```python
from build123d import *

# Parameters (mm, degrees)
SKETCH1_W           = 40
SKETCH1_H           = 25
BOSS_EXTRUDE1_DEPTH = 14
SKETCH2_R           = 8.15
CUT_EXTRUDE1_DEPTH  = 10.3
CUT_EXTRUDE2_REACH  = 50.281
SKETCH3_R           = 2.65
CUT_EXTRUDE3_REACH  = 51.204
SKETCH4_R           = 1.5
CHAMFER1_SIZE       = 5


with BuildPart() as part:
    # Sketch1 → Boss-Extrude1 (new body)
    with BuildSketch(Plane.XY):
        with Locations((20, 12.5)):
            Rectangle(SKETCH1_W, SKETCH1_H)
    extrude(amount=BOSS_EXTRUDE1_DEPTH)

    # Sketch2 → Cut-Extrude1 (cut)
    with BuildSketch(Plane.XY.offset(14)):
        with Locations((20, 12.5)):
            Circle(SKETCH2_R)
    extrude(amount=-CUT_EXTRUDE1_DEPTH, mode=Mode.SUBTRACT)

    # Sketch3 → Cut-Extrude2 (cut, up to next)
    with BuildSketch(Plane.XY.offset(3.7), mode=Mode.PRIVATE) as cut_extrude2_sk1:
        with Locations((20, 12.5)):
            Circle(SKETCH3_R)
    cut_extrude2_tool1 = extrude(cut_extrude2_sk1.sketch, amount=-CUT_EXTRUDE2_REACH, mode=Mode.PRIVATE) & part.part
    add(cut_extrude2_tool1.solids().sort_by_distance((20, 12.5, 3.7))[0], mode=Mode.SUBTRACT)

    # Sketch4 → Cut-Extrude3 (cut, up to next)
    with BuildSketch(Plane.XY.offset(14), mode=Mode.PRIVATE) as cut_extrude3_sk1:
        with Locations((6, 12.5)):
            Circle(SKETCH4_R)
    cut_extrude3_tool1 = extrude(cut_extrude3_sk1.sketch, amount=-CUT_EXTRUDE3_REACH, mode=Mode.PRIVATE) & part.part
    # Sketch4 → Cut-Extrude3 (cut, up to next)
    with BuildSketch(Plane.XY.offset(14), mode=Mode.PRIVATE) as cut_extrude3_sk2:
        with Locations((34, 12.5)):
            Circle(SKETCH4_R)
    cut_extrude3_tool2 = extrude(cut_extrude3_sk2.sketch, amount=-CUT_EXTRUDE3_REACH, mode=Mode.PRIVATE) & part.part
    add(cut_extrude3_tool1.solids().sort_by_distance((6, 12.5, 14))[0], mode=Mode.SUBTRACT)
    add(cut_extrude3_tool2.solids().sort_by_distance((34, 12.5, 14))[0], mode=Mode.SUBTRACT)

    # Chamfer1
    chamfer1_edges = [part.edges().sort_by_distance(p)[0] for p in [
        (0, 25, 7),
        (40, 25, 7),
        (40, 0, 7),
        (0, 0, 7),
    ]]
    chamfer(chamfer1_edges, length=CHAMFER1_SIZE)


solid = part.part
```
Here's how the part is built. I have some questions about the finished solid (model axes, mm). A direction names the side the tool comes from. Give positions to 0.01 mm unless a question says otherwise; leave off trailing zeros. Order: outer loops, then holes, each group sorted by start corner. A loop starts at its lowest first (then second) coordinate and runs counter-clockwise, first axis right, second up. Notation, with made-up numbers: M -11,1.25 L 22,1.25 A36 cw 22,36.25 Z; hole C -28.5,-7 d2. An arc over 180 degrees is marked long. Use a Markdown table: item, result. Add a question column.
1. If we mould it in two halves opening along X, with no side actions, what happens to faces 1 (the cylindrical face through (22.45, 11.49, 1.88)), 2 (the flat face through (20, 0, 7)), 3 (the flat face through (40, 12, 7))? For each: +X half, -X half, draft (parallel to the pull), parting line (faces both ways), or undercut.
2. On a 3-axis mill with a long thin cutter (end or side, diameter ignored), from which of +Z, -Z, +X, -X, +Y, -Y can I reach the whole of each face in a straight line? I mean faces 4 (the flat face through (3, 2, 7)), 5 (the cylindrical face through (11.858, 12.858, 8.922)). Say none if no direction works.
3. Suppose I cut it at D-D (x = 20). List the corners of the cut face in (y, z) for me.
4. I need wall thicknesses on probe 1 along Y at (x, z) = (20, 10); probe 2 along Y at (x, z) = (34, 5.25); probe 3 along X at (y, z) = (15.75, 10). Which ranges of each line are inside material? Lowest first, please. Write a range as from..to.
5. Suppose I cut it at B-B (z = 2). List the corners of the cut face in (x, y) for me.
6. For pin 1 Ø2 at (x, y) = (17, 10.5) entering from -Z; pin 2 Ø1.5 at (y, z) = (4, 10) entering from +X; pin 3 Ø8.5 at (x, y) = (20, 12.5) entering from +Z; pin 4 Ø2.5 at (x, y) = (34, 12.5) entering from +Z, each with a flat end and sliding along its axis, tell me the tip position at first contact or that it passes through.
7. Suppose I cut it at A-A (x = 34). List the corners of the cut face in (y, z) for me, and give its area (3 significant figures).
8. Suppose I cut it at C-C (y = 12.5). List the corners of the cut face in (x, z) for me, and give its area (4 significant figures).
Results list:
| question | item | result |
|---|---|---|
| 1 | face 1 | undercut |
| 1 | face 2 | draft |
| 1 | face 3 | +X half |
| 2 | face 4 | +Z, -Z, -X, -Y |
| 2 | face 5 | +Z |
| 3 | outline | M 0,0 L 9.85,0 L 9.85,3.7 L 4.35,3.7 L 4.35,14 L 0,14 Z; M 15.15,0 L 25,0 L 25,14 L 20.65,14 L 20.65,3.7 L 15.15,3.7 Z |
| 4 | probe 1 | y = 0..4.35, 20.65..25 |
| 4 | probe 2 | y = 0..11, 14..25 |
| 4 | probe 3 | x = 0..12.53, 27.47..40 |
| 5 | outline | M 0,5 L 5,0 L 35,0 L 40,5 L 40,20 L 35,25 L 5,25 L 0,20 Z; hole C 6,12.5 d3; hole C 20,12.5 d5.3; hole C 34,12.5 d3 |
| 6 | pin 1 | stops at z = 0 |
| 6 | pin 2 | stops at x = 39.75 |
| 6 | pin 3 | stops at z = 3.7 |
| 6 | pin 4 | passes through |
| 7 | outline | M 0,0 L 11,0 L 11,14 L 0,14 Z; M 14,0 L 25,0 L 25,14 L 14,14 Z |
| 7 | area | 308 mm² |
| 8 | outline | M 0,0 L 4.5,0 L 4.5,14 L 0,14 Z; M 7.5,0 L 17.35,0 L 17.35,3.7 L 11.85,3.7 L 11.85,14 L 7.5,14 Z; M 22.65,0 L 32.5,0 L 32.5,14 L 28.15,14 L 28.15,3.7 L 22.65,3.7 Z; M 35.5,0 L 40,0 L 40,14 L 35.5,14 Z |
| 8 | area | 288.5 mm² |
